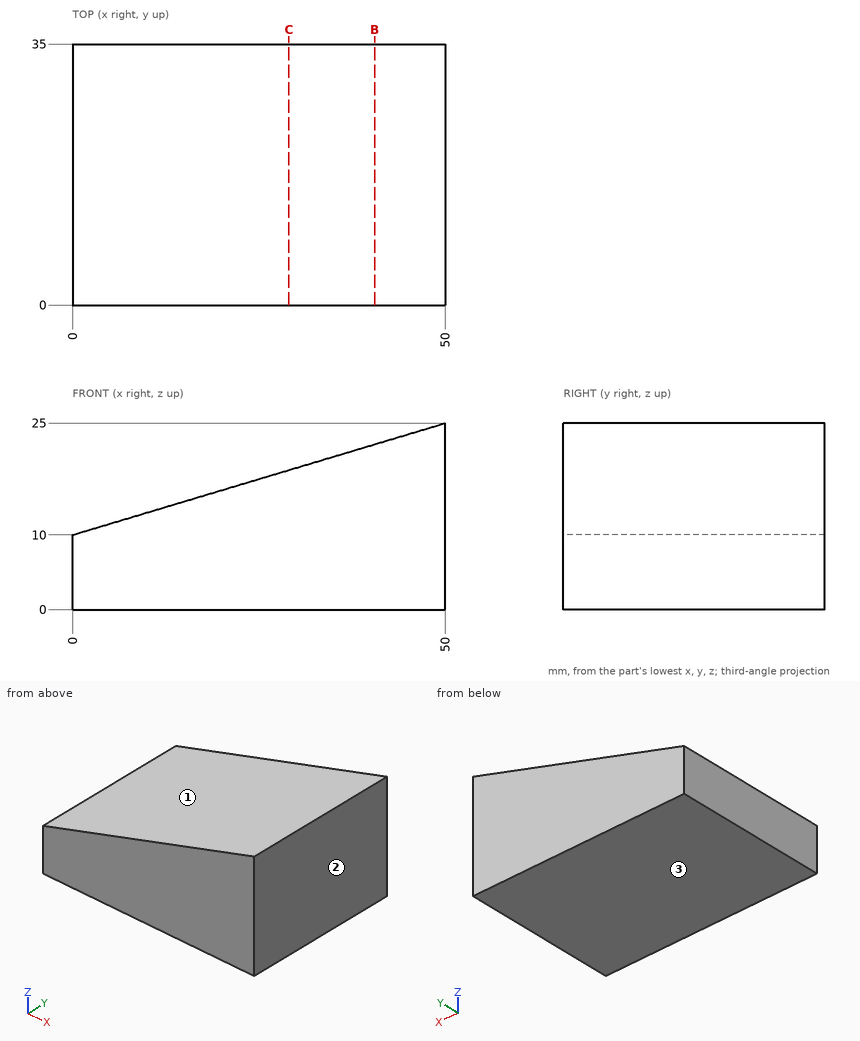
Geometry: see drawing. Coordinates: mm, zero at the bounding-box minimum. Coordinates: 2 decimals unless noted, no trailing zeros. Order: outer loops, then holes, each group sorted by start corner. A loop starts at its lowest first (then second) coordinate and runs counter-clockwise, first axis right, second up. Notation, with made-up numbers: M -22,1 L 31,1 A28 ccw 31,36 Z; hole C -13.75,5 d10. An arc over 180 degrees is marked long. Write item = value, one per line. Start each with the question number.
(1) First-contact query: P1, Ø3, axis at x = 11.5, y = 29.5, coming from the +Z side; P2, Ø1, axis at x = 16, y = 17, coming from the +Z side; P3, Ø4, axis at x = 5, y = 6, coming from the +Z side. Flat tips, straight axial feed; report the tip coordinate or a pass-through.
(2) Section B-B on x = 40.5. Output: boundary loops of the cut face in (y, z), and give its area (3 significant figures).
(3) Section C-C on x = 29. Output: boundary loops of the cut face in (y, z), and give its area (4 significant figures).
(4) Pull-direction query (Z, two-part tool) for the marked faces 1, 2 and 3; classes: released by +Z, released by -Z, zero draft, split by the parting line, or undercut.
(5) Line query: line 1 along Z through (x, y) = (24.5, 16.5); line 2 along Z through (x, y) = (37, 17). Output: solid intervals per line, ascending. Write a range as [from, to].
Result set:
q1.P1 = 13.9
q1.P2 = 14.95
q1.P3 = 12.1
q2.outline = M 0,0 L 35,0 L 35,22.15 L 0,22.15 Z
q2.area = 775 mm²
q3.outline = M 0,0 L 35,0 L 35,18.7 L 0,18.7 Z
q3.area = 654.5 mm²
q4.face_1 = released by +Z
q4.face_2 = zero draft
q4.face_3 = released by -Z
q5.line_1 = [0, 17.35]
q5.line_2 = [0, 21.1]
